Here's the drawing with two shaded views (mm, measured from the low corner). I have some questions. A direction names the side the tool comes from. Round coordinates to 2 decimals unless told otherwise and drop trailing zeros. Write each loop counter-clockwise with the first axis right and the second up, starting at its lowest first coordinate (ties: lowest second). Pieces come first, ordered by that corner, then holes. Notation, with made-up numbers: M -25,57.5 L 16,57.5 A18 cw 16,92.5 Z; hole C 15,15 d8. An arc over 180 degrees is marked long. Answer as a JSON object with one key per item and string values. Group by question number.
1) I'm going to push flat-ended pins straight in: pin 1 Ø2 at (x, y) = (0.5, 20.5) entering from -Z; pin 2 Ø10 at (x, y) = (28, 22) entering from -Z. Where does each tip first touch, or does it pass through?
2) Suppose I cut it at A-A, the plane z = 15.25. Write out the boundary of the cut face in (x, y), and give its area (3 significant figures).
3) Please list where these lines run through material, in increasing order: L1, parallel to Y at x = 20, z = 16.25; L2, parallel to Z at x = 16, y = 6.5. Write a range as [from, to].
4) If we mould it in two halves opening along Y, with no side actions, what happens to the marked faces 3, 4 and 5? For each: +Y half, -Y half, draft (parallel to the pull), parting line (faces both ways), or undercut.
5) On a 3-axis mill with a long thin cutter (end or side, diameter ignored), from which of +Z, -Z, +X, -X, +Y, -Y can I reach the whole of each face in a straight line? I mean the marked faces 1 and 2. Say none if no direction works.
6) Suppose I cut it at B-B, the plane x = 3.5. Write out the boundary of the cut face in (y, z), and give its area (3 significant figures).
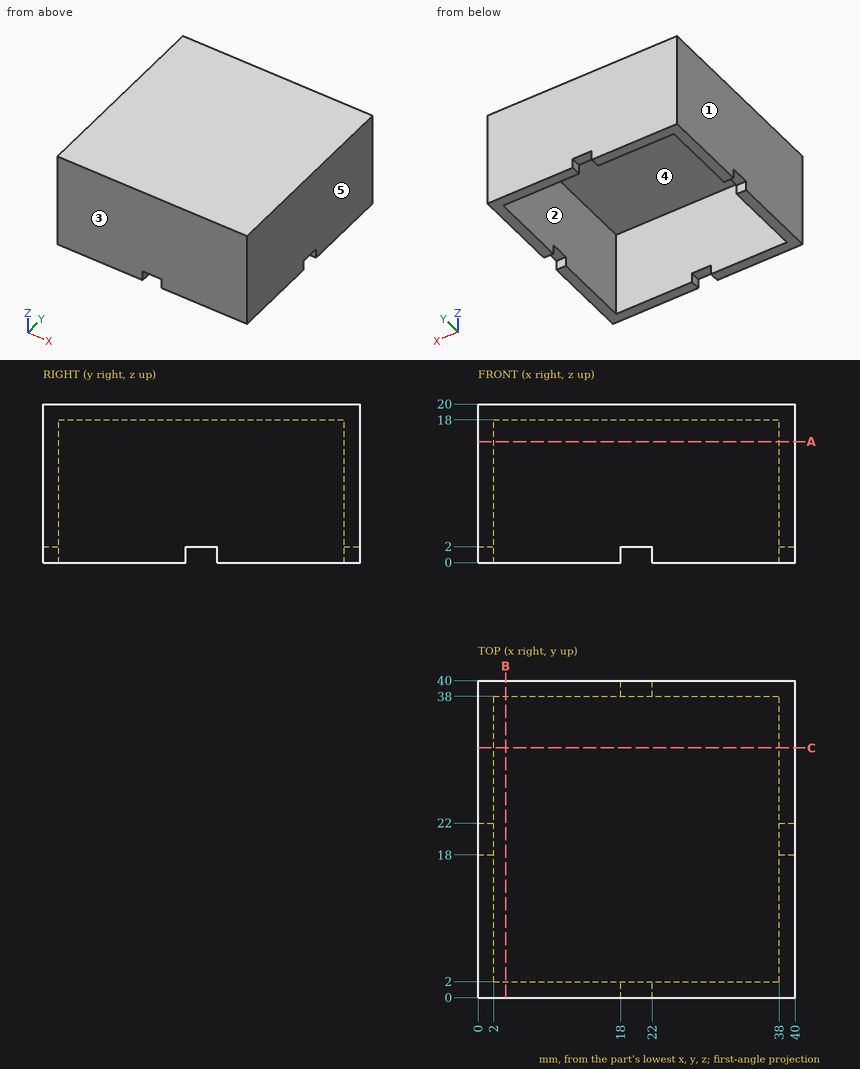
Results:
{
 "1": {"pin 1": "z = 2", "pin 2": "z = 18"},
 "2": {"outline": "M 0,0 L 40,0 L 40,40 L 0,40 Z; hole M 2,2 L 38,2 L 38,38 L 2,38 Z", "area": "304 mm^2"},
 "3": {"L1": "[0, 2], [38, 40]", "L2": "[18, 20]"},
 "4": {"face 3": "-Y half", "face 4": "undercut", "face 5": "draft"},
 "5": {"face 1": "+Z, -Z, -X, +Y, -Y", "face 2": "-Z"},
 "6": {"outline": "M 0,0 L 2,0 L 2,18 L 38,18 L 38,0 L 40,0 L 40,20 L 0,20 Z", "area": "152 mm^2"}
}
